Verification items for this drawing (mm, ordinates from the low corner). Give positions to 0.01 mm unless a question says otherwise; leave off trailing zeros. Loops run counter-clockwise (first coordinate to the right, second up) from the corner with the lowest first, then second, coordinate; pieces in that order, holes last. Notation, with made-up numbers: M 13.5,9 L 40.5,9 A32 cw 40.5,37 Z; hole C -25.75,33.5 d9. An arc over 180 degrees is marked long. Answer in a Markdown table with one row per item.
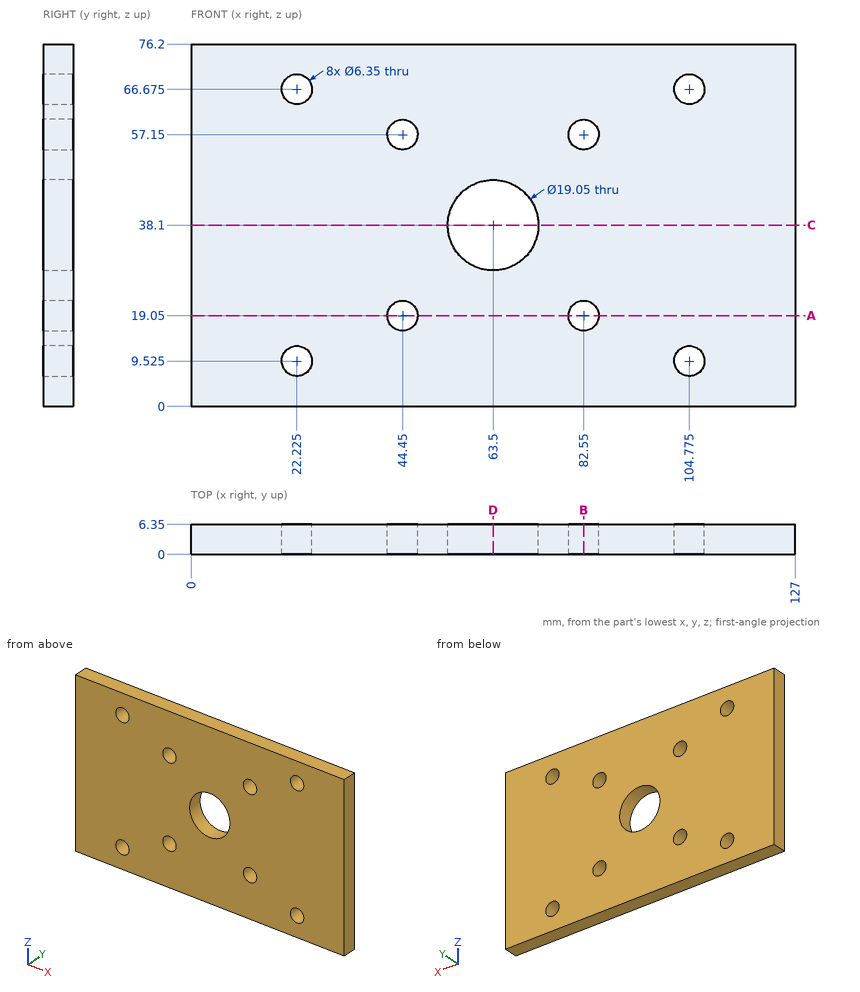
Item 1: Sectioned sample at A-A (z = 19.05). Record the cut outline in (x, y) (3 decimals).
Reported:
| item | result |
|---|---|
| outline | M 0,0 L 41.275,0 L 41.275,6.35 L 0,6.35 Z; M 47.625,0 L 79.375,0 L 79.375,6.35 L 47.625,6.35 Z; M 85.725,0 L 127,0 L 127,6.35 L 85.725,6.35 Z |
Item 2: Go/stop test with a flat-tipped pin: pin 1 (11.5 mm diameter, centred on x = 63.5, z = 38.1, fed in from +Y). Record where the tip stops, or that it passes through.
Reported:
| item | result |
|---|---|
| pin 1 | passes through |
Item 3: Sectioned sample at C-C (z = 38.1). Record the cut outline in (x, y) (3 decimals), and give its area (3 significant figures).
Reported:
| item | result |
|---|---|
| outline | M 0,0 L 53.975,0 L 53.975,6.35 L 0,6.35 Z; M 73.025,0 L 127,0 L 127,6.35 L 73.025,6.35 Z |
| area | 685 mm^2 |
Item 4: Sectioned sample at B-B (x = 82.55). Record the cut outline in (y, z) (3 decimals), and give its area (3 significant figures).
Reported:
| item | result |
|---|---|
| outline | M 0,0 L 6.35,0 L 6.35,15.875 L 0,15.875 Z; M 0,22.225 L 6.35,22.225 L 6.35,53.975 L 0,53.975 Z; M 0,60.325 L 6.35,60.325 L 6.35,76.2 L 0,76.2 Z |
| area | 403 mm^2 |
Item 5: Scan lines: L1, parallel to X at y = 4.5, z = 19.05 (3 decimals); L2, parallel to X at y = 1, z = 10; L3, parallel to Z at x = 43.5, y = 4.5. Record each from-to range of solid material in increasing order. Write a range as [from, to].
Reported:
| item | result |
|---|---|
| L1 | x = [0, 41.275], [47.625, 79.375], [85.725, 127] |
| L2 | x = [0, 19.09], [25.36, 101.64], [107.91, 127] |
| L3 | z = [0, 16.02], [22.08, 54.12], [60.18, 76.2] |
Item 6: Sectioned sample at D-D (x = 63.5). Record the cut outline in (y, z) (3 decimals), and give its area (3 significant figures).
Reported:
| item | result |
|---|---|
| outline | M 0,0 L 6.35,0 L 6.35,28.575 L 0,28.575 Z; M 0,47.625 L 6.35,47.625 L 6.35,76.2 L 0,76.2 Z |
| area | 363 mm^2 |
